from build123d import *

# Parameters (mm, degrees)
F0_W      = 875
F0_H      = 22
F1_DEPTH  = 31
F2_T      = -2
F3_R      = 5
F4_DEPTH  = 61
F5_W      = 16
F5_H      = 16
F6_DEPTH  = 46
F7_R      = 8
F8_DEPTH  = 96
F9_R      = 10
F10_W     = 27
F10_H     = 21.5130257002
F11_DEPTH = 25
F12_W     = 27
F12_H     = 18.3594822884
F13_DEPTH = 25


with BuildPart() as f1:
    # F0 (on Right) → F1 (new body)
    with BuildSketch(Plane.YZ):
        with Locations((49.2357180723, -11)):
            Rectangle(F0_W, F0_H)
    extrude(amount=-F1_DEPTH)

    # F2
    f2_openings = [f1.faces().sort_by_distance(p)[0] for p in [
        (-15.5, 49.235718, 0),
    ]]
    offset(amount=F2_T, openings=f2_openings)

    # F3 (on face) → F4 (cut)
    with BuildSketch(Plane.YZ):
        with Locations((478.7357180723, -11)):
            Circle(F3_R)
    extrude(amount=-F4_DEPTH, mode=Mode.SUBTRACT)

    # F5 (on face) → F6 (cut)
    with BuildSketch(Plane.XY):
        with Locations((-18, 478.7357180723)):
            Rectangle(F5_W, F5_H)
    extrude(amount=-F6_DEPTH, mode=Mode.SUBTRACT)

    # F7 (on face) → F8 (cut)
    with BuildSketch(Plane.YZ):
        with Locations((-376.4913082123, -11)):
            Circle(F7_R)
        with Locations((-281.4913082123, -11)):
            Circle(F7_R)
    extrude(amount=-F8_DEPTH, mode=Mode.SUBTRACT)

    # F9
    f9_edges = [f1.edges().sort_by_distance(p)[0] for p in [
        (-5, 486.735718, 0),
        (-28.5, 486.735718, 0),
        (-6, 484.735718, -20),
        (-5, 486.735718, -22),
        (-27.5, 484.735718, -20),
        (-28.5, 486.735718, -22),
    ]]
    fillet(f9_edges, radius=F9_R)

    # F10 (on face) → F11 (cut)
    with BuildSketch(Plane.XY.offset(-20)):
        with Locations((-15.5, 481.4922309224)):
            Rectangle(F10_W, F10_H)
    extrude(amount=-F11_DEPTH, mode=Mode.SUBTRACT)

    # F12 (on face) → F13 (cut)
    with BuildSketch(Plane.XY.offset(-20)):
        with Locations((-15.5, 482.3970198631)):
            Rectangle(F12_W, F12_H)
    extrude(amount=F13_DEPTH, mode=Mode.SUBTRACT)


solid = f1.part
Input: part model. Units: mm. Frame: model coordinates. A direction names the side the tool comes from. Coordinates: 2 decimals unless noted, no trailing zeros. Loops run counter-clockwise (first coordinate to the right, second up) from the corner with the lowest first, then second, coordinate; pieces in that order, holes last. Notation, with made-up numbers: (81.25, 8) -> (88.25, 8) arc R33 cw to (88.25, 42) -> close; hole circle Ø2 at (-25, 43). An arc over 180 degrees is marked (long way). One line per item, written item: value.
(1) Ray query, line 1 along X through (y, z) = (263.5, -8.5); line 2 along Z through (x, y) = (-22, -56); line 3 along Y through (x, z) = (-15, -6). Return the intervals inside material, ascending.
Answer below:
line 1: x = -31 to -29, -2 to 0
line 2: z = -22 to -20
line 3: y = -388.26 to -386.26
(2) Draft query along Z for faces 1 (the face through (-15, 38, -22)), 2 (the face through (-29.986, -384.484, -10.648)), 3 (the face through (-1.6, 42.2, 0)). Return one class per face: pulls with the +Z half, pulls with the -Z half, needs draft (parallel to the pull), parting line crosses it, or undercut.
Answer below:
face 1: pulls with the -Z half
face 2: undercut
face 3: pulls with the +Z half
(3) Pin query (flat end, axial travel): pin 1 Ø8 at (y, z) = (478.74, -11) entering from -X; pin 2 Ø4 at (x, z) = (-8, -4) entering from +Y; pin 3 Ø13.5 at (x, y) = (-12, 225) entering from +Z; pin 4 Ø0.6 at (x, z) = (-20.5, -21) entering from +Y. Return the tip coordinate at first contact, or that it passes through.
Answer below:
pin 1: passes through
pin 2: stops at y = -386.26
pin 3: stops at z = -20
pin 4: stops at y = 470.74
(4) Cut plane B-B (y = 259.5). Output: boundary loops of the cut face in (x, z).
Answer below:
outline: (-31, -22) -> (0, -22) -> (0, 0) -> (-2, 0) -> (-2, -20) -> (-29, -20) -> (-29, 0) -> (-31, 0) -> close
(5) Set-up query: faces 4 (the face through (-0.986, -384.484, -10.648)), 5 (the face through (-15, -386.264, -10)). Return all of +Z, -Z, +X, -X, +Y, -Y with unobstructed straight access to the full face (end or side cutting, diameter ignored); none if empty.
Answer below:
face 4: +X, -X
face 5: +Z, +Y
(6) Cut plane A-A (x = -21). Output: boundary loops of the cut face in (y, z), then the cut area to 3 significant figures.
Answer below:
outline: (-388.26, -22) -> (470.74, -22) -> (470.74, -20) -> (-386.26, -20) -> (-386.26, 0) -> (-388.26, 0) -> close
area: 1,760 mm2
